Check sheet for the modelled part. Datum: model origin and axes. Units: mm. Round coordinates to 2 decimals unless told otherwise and drop trailing zeros. Order: outer loops, then holes, each group sorted by start corner. A loop starts at its lowest first (then second) coordinate and runs counter-clockwise, first axis right, second up.
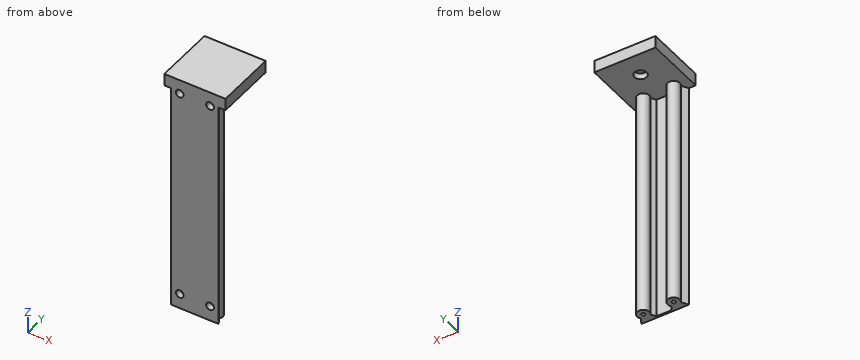
```python
from build123d import *

# Parameters (mm, degrees)
SKETCH1_R           = 5
BOSS_EXTRUDE1_DEPTH = 220
BOSS_EXTRUDE4_DEPTH = 220
SKETCH5_R           = 1.37
CUT_EXTRUDE1_DEPTH  = 7
SKETCH6_R           = 1.37
CUT_EXTRUDE2_DEPTH  = 7
CUT_EXTRUDE4_DEPTH  = 10.8
CUT_EXTRUDE5_DEPTH  = 10.8
SKETCH11_R          = 2
CUT_EXTRUDE6_DEPTH  = 7
SKETCH12_R          = 1.5
CUT_EXTRUDE7_DEPTH  = 7
SKETCH13_W          = 50
SKETCH13_H          = 50
BOSS_EXTRUDE5_DEPTH = 10
SKETCH14_R          = 5
CUT_EXTRUDE8_DEPTH  = 5
SKETCH4_2_R         = 3.2
CUT_EXTRUDE9_DEPTH  = 5


with BuildPart() as part:
    # Sketch1 → Boss-Extrude1 (new body)
    with BuildSketch(Plane.XY):
        Circle(SKETCH1_R)
        with BuildLine():
            Line((-4, -3), (-7, -8.196152423))
            Line((-7, -8.196152423), (7, -8.196152423))
            Line((7, -8.196152423), (4, -3))
            ThreePointArc((4, -3), (0, 5), (-4, -3))
        make_face()
        with BuildLine():
            Line((28.8, -3), (31.8, -8.196152423))
            Line((31.8, -8.196152423), (17.8, -8.196152423))
            Line((17.8, -8.196152423), (20.8, -3))
            ThreePointArc((20.8, -3), (24.8, 5), (28.8, -3))
        make_face()
    extrude(amount=BOSS_EXTRUDE1_DEPTH)

    # Sketch3 → Boss-Extrude4 (add)
    with BuildSketch(Plane.XY.offset(220)):
        Polygon((7, -8.196152423), (17.8, -8.196152423), (18.65, -8.196152423), (18.65, -6.723909236), (6.15, -6.723909236), (6.15, -8.196152423), align=None)
    extrude(amount=-BOSS_EXTRUDE4_DEPTH)

    # Sketch5 → Cut-Extrude1 (cut)
    with BuildSketch(Plane(origin=(0, 0, 0), x_dir=(-1, 0, 0), z_dir=(0, 0, -1))):
        Circle(SKETCH5_R)
        with Locations((-24.8, 0)):
            Circle(SKETCH5_R)
    extrude(amount=-CUT_EXTRUDE1_DEPTH, mode=Mode.SUBTRACT)

    # Sketch6 → Cut-Extrude2 (cut)
    with BuildSketch(Plane.XY.offset(220)):
        Circle(SKETCH6_R)
        with Locations((24.8, 0)):
            Circle(SKETCH6_R)
    extrude(amount=-CUT_EXTRUDE2_DEPTH, mode=Mode.SUBTRACT)

    # Sketch9 → Cut-Extrude4 (cut)
    with BuildSketch(Plane(origin=(0, 0, 0), x_dir=(-1, 0, 0), z_dir=(0, 0, -1))):
        with BuildLine():
            Line((-28.8, -3), (-31.8, -8.196152423))
            Line((-31.8, -8.196152423), (7, -8.196152423))
            Line((7, -8.196152423), (4, -3))
            ThreePointArc((4, -3), (0, 5), (-4, -3))
            Line((-4, -3), (-6.15, -6.723909236))
            Line((-6.15, -6.723909236), (-18.65, -6.723909236))
            Line((-18.65, -6.723909236), (-20.8, -3))
            ThreePointArc((-20.8, -3), (-24.8, 5), (-28.8, -3))
        make_face()
    extrude(amount=-CUT_EXTRUDE4_DEPTH, mode=Mode.SUBTRACT)

    # Sketch10 → Cut-Extrude5 (cut)
    with BuildSketch(Plane.XY.offset(220)):
        with BuildLine():
            Line((20.8, -3), (18.65, -6.723909236))
            Line((18.65, -6.723909236), (6.15, -6.723909236))
            Line((6.15, -6.723909236), (4, -3))
            ThreePointArc((4, -3), (0, 5), (-4, -3))
            Line((-4, -3), (-7, -8.196152423))
            Line((-7, -8.196152423), (31.8, -8.196152423))
            Line((31.8, -8.196152423), (28.8, -3))
            ThreePointArc((28.8, -3), (24.8, 5), (20.8, -3))
        make_face()
    extrude(amount=-CUT_EXTRUDE5_DEPTH, mode=Mode.SUBTRACT)

    # Sketch11 → Cut-Extrude6 (cut)
    with BuildSketch(Plane.XY.offset(209.2)):
        Circle(SKETCH11_R)
        with Locations((24.8, 0)):
            Circle(SKETCH11_R)
    extrude(amount=-CUT_EXTRUDE6_DEPTH, mode=Mode.SUBTRACT)

    # Sketch12 → Cut-Extrude7 (cut)
    with BuildSketch(Plane(origin=(0, 0, 10.8), x_dir=(-1, 0, 0), z_dir=(0, 0, -1))):
        Circle(SKETCH12_R)
        with Locations((-24.8, 0)):
            Circle(SKETCH12_R)
    extrude(amount=-CUT_EXTRUDE7_DEPTH, mode=Mode.SUBTRACT)

    # Sketch13 → Boss-Extrude5 (add)
    with BuildSketch(Plane.XY.offset(209.2)):
        with Locations((12.4, 16.803847577)):
            Rectangle(SKETCH13_W, SKETCH13_H)
    extrude(amount=-BOSS_EXTRUDE5_DEPTH)

    # Sketch14 → Cut-Extrude8 (cut)
    with BuildSketch(Plane(origin=(0, 0, 199.2), x_dir=(-1, 0, 0), z_dir=(0, 0, -1))):
        with Locations((-12.4, 22.303847577)):
            Circle(SKETCH14_R)
    extrude(amount=-CUT_EXTRUDE8_DEPTH, mode=Mode.SUBTRACT)

    # Sketch4_2 → Cut-Extrude9 (cut)
    with BuildSketch(Plane.XZ.offset(8.196152423)):
        with Locations((24.8, 197.5)):
            Circle(SKETCH4_2_R)
        with Locations((24.8, 23.2)):
            Circle(SKETCH4_2_R)
        with Locations((0, 23.2)):
            Circle(SKETCH4_2_R)
        with Locations((0, 197.5)):
            Circle(SKETCH4_2_R)
    extrude(amount=-CUT_EXTRUDE9_DEPTH, mode=Mode.SUBTRACT)


solid = part.part
```
Item 1: Sectioned sample at C-C (y = 25). Record the cut outline in (x, z), and give its area (3 significant figures).
Answer:
outline: (-12.6, 199.2) - (8.19, 199.2) - (8.19, 204.2) - (16.61, 204.2) - (16.61, 199.2) - (37.4, 199.2) - (37.4, 209.2) - (-12.6, 209.2) - close
area: 458 mm2
Item 2: Sectioned sample at B-B (x = 12.4). Record the cut outline in (y, z), and give its area (3 significant figures).
Answer:
outline: (-8.2, 10.8) - (-6.72, 10.8) - (-6.72, 199.2) - (17.3, 199.2) - (17.3, 204.2) - (27.3, 204.2) - (27.3, 199.2) - (41.8, 199.2) - (41.8, 209.2) - (-8.2, 209.2) - close
area: 727 mm2
Item 3: Sectioned sample at A-A (z = 23.2). Record the cut outline in (x, y), and give its area (3 significant figures).
Answer:
outline: (-7, -8.2) - (-3.2, -8.2) - (-3.2, -3.2) - (3.2, -3.2) - (3.2, -8.2) - (21.6, -8.2) - (21.6, -3.2) - (28, -3.2) - (28, -8.2) - (31.8, -8.2) - (28.8, -3) arc R5 ccw (long way) to (20.8, -3) - (18.65, -6.72) - (6.15, -6.72) - (4, -3) arc R5 ccw (long way) to (-4, -3) - close
area: 202 mm2
Item 4: Go/stop test with flat-tipped pins: P1, Ø4, axis at x = 24.8, z = 23.2, coming from the -Y side; P2, Ø8, axis at x = 22.5, z = 91, coming from the +Y side; P3, Ø4, axis at x = 15.5, y = 1, coming from the -Z side. Record where each tip stops, or that it passes through.
Answer:
P1: stops at y = -3.2
P2: stops at y = 5
P3: stops at z = 199.2
Item 5: Sectioned sample at D-D (z = 87.5). Record the cut outline in (x, y).
Answer:
outline: (-7, -8.2) - (31.8, -8.2) - (28.8, -3) arc R5 ccw (long way) to (20.8, -3) - (18.65, -6.72) - (6.15, -6.72) - (4, -3) arc R5 ccw (long way) to (-4, -3) - close
Item 6: Scan lines: line 1 along Y through (x, z) = (24.8, 15.5); line 2 along Z through (x, y) = (12, 1); line 3 along X through (y, z) = (4.5, 195). Record each from-to range of solid material in increasing order.
Answer:
line 1: y = -8.2 to -1.5, 1.5 to 5
line 2: z = 199.2 to 209.2
line 3: x = -2.18 to 2.18, 22.62 to 26.98
